Part model, mm, in its own coordinate system. A direction names the side the tool comes from. Round coordinates to 2 decimals unless told otherwise and drop trailing zeros. Loops run counter-clockwise (first coordinate to the right, second up) from the corner with the lowest first, then second, coordinate; pieces in that order, holes last.
from build123d import *

# Parameters (mm, degrees)
F0_W      = 50.8
F0_H      = 50.8
F1_DEPTH  = 50.8
F2_R      = 10.16
F3_DEPTH  = 2.54
F4_W      = 25.4
F4_H      = 14.759139
F5_DEPTH  = 2.54
F6_W      = 7.62
F6_H      = 2.876111
F7_DEPTH  = 5.08
F8_R      = 3.81
F9_DEPTH  = 5.08
F10_R     = 1.905
F11_DEPTH = 20.32
F12_R     = 1.778
F14_DEPTH = 53.34
F15_SIZE  = 1.27


with BuildPart() as f1:
    # F0 (on Front) → F1 (new body)
    with BuildSketch(Plane.XZ):
        with Locations((25.4, 25.4)):
            Rectangle(F0_W, F0_H)
    extrude(amount=F1_DEPTH)

    # F2 (on Right) → F3 (join)
    with BuildSketch(Plane.YZ):
        with Locations((-25.4, 35.56)):
            Circle(F2_R)
    extrude(amount=-F3_DEPTH)

    # F4 (on Right) → F5 (join)
    with BuildSketch(Plane.YZ):
        with Locations((-25.4, 10.40043)):
            Rectangle(F4_W, F4_H)
    extrude(amount=-F5_DEPTH)

    # F6 (on Right) → F7 (cut)
    with BuildSketch(Plane.YZ):
        with Locations((-19.05, 13.801944)):
            Rectangle(F6_W, F6_H)
        with Locations((-31.75, 13.801944)):
            Rectangle(F6_W, F6_H)
    extrude(amount=-F7_DEPTH, mode=Mode.SUBTRACT)

    # F8 (on Right) → F9 (join)
    with BuildSketch(Plane.YZ):
        with Locations((-25.4, 8.100861)):
            Circle(F8_R)
    extrude(amount=-F9_DEPTH)

    # F10 (on Right) → F11 (cut)
    with BuildSketch(Plane.YZ):
        with Locations((-31.771343, 38.1)):
            Circle(F10_R)
        with Locations((-19.028657, 38.1)):
            Circle(F10_R)
        with Locations((-19.028657, 33.02)):
            Circle(F10_R)
        with Locations((-31.771343, 33.02)):
            Circle(F10_R)
    extrude(amount=-F11_DEPTH, mode=Mode.SUBTRACT)

    # F12
    f12_edges = [f1.edges().sort_by_distance(p)[0] for p in [
        (0, -50.8, 25.4),
        (25.4, -50.8, 0),
        (50.8, -50.8, 25.4),
        (25.4, -50.8, 50.8),
        (50.8, -25.4, 50.8),
        (0, -25.4, 50.8),
        (25.4, 0, 50.8),
        (50.8, -25.4, 0),
        (50.8, 0, 25.4),
        (0, 0, 25.4),
        (25.4, 0, 0),
        (0, -25.4, 0),
    ]]
    fillet(f12_edges, radius=F12_R)

    # F13 (on Top) → F14 (join)
    with BuildSketch(Plane.XY):
        Polygon((18.288, -8.128), (8.128, -8.128), (8.128, -42.672), (42.672, -42.672), (42.672, -8.128), (32.512, -8.128), (32.512, -17.272), (18.288, -17.272), align=None)
    extrude(amount=F14_DEPTH)

    # F15
    f15_edges = [f1.edges().sort_by_distance(p)[0] for p in [
        (13.208, -8.128, 53.34),
        (8.128, -25.4, 53.34),
        (25.4, -42.672, 53.34),
        (42.672, -25.4, 53.34),
        (37.592, -8.128, 53.34),
        (32.512, -12.7, 53.34),
        (25.4, -17.272, 53.34),
        (18.288, -12.7, 53.34),
    ]]
    chamfer(f15_edges, length=F15_SIZE)


solid = f1.part
1) Tool access for faces 4 (the face through (-1, -38.1, 10)), 5 (the face through (25.73, -0.53, 0.51)), 6 (the face through (-1, -32, 15.24)): list every direction of +Z, -Z, +X, -X, +Y, -Y with a clear straight run to the whole face (end or side of a thin tool).
Values:
face 4: +Z, -Z, -X, -Y
face 5: -Z, +X, -X, +Y
face 6: -X
2) Slice it at D-D, the plane z = 47. Give the cut face in (x, y).
Values:
outline: (0, -49.02) arc R1.78 ccw to (1.78, -50.8) - (49.02, -50.8) arc R1.78 ccw to (50.8, -49.02) - (50.8, -1.78) arc R1.78 ccw to (49.02, 0) - (1.78, 0) arc R1.78 ccw to (0, -1.78) - close
3) Slice it at B-B, the plane y = -25.4. Give the cut face in (x, z).
Values:
outline: (-5.08, 4.29) - (-2.54, 4.29) - (-2.54, 3.02) - (0, 3.02) - (0, 1.78) arc R1.78 ccw to (1.78, 0) - (49.02, 0) arc R1.78 ccw to (50.8, 1.78) - (50.8, 49.02) arc R1.78 ccw to (49.02, 50.8) - (42.67, 50.8) - (42.67, 52.07) - (41.4, 53.34) - (9.4, 53.34) - (8.13, 52.07) - (8.13, 50.8) - (1.78, 50.8) arc R1.78 ccw to (0, 49.02) - (0, 45.72) - (-2.54, 45.72) - (-2.54, 25.4) - (0, 25.4) - (0, 17.78) - (-2.54, 17.78) - (-2.54, 11.91) - (-5.08, 11.91) - close
4) Wall check: line 1 along X through (y, z) = (-37, 36); line 2 along Y through (x, z) = (-1, 38). Give the ranges that are in metal, low to high.
Values:
line 1: x = 0 to 50.8
line 2: y = -35.26 to -33.67, -29.87 to -20.93, -17.13 to -15.54
5) Slice it at A-A, the plane z = 16.5. Give the cut face in (x, y), then the cut area to 3 significant figures.
Values:
outline: (-2.54, -38.1) - (0, -38.1) - (0, -49.02) arc R1.78 ccw to (1.78, -50.8) - (49.02, -50.8) arc R1.78 ccw to (50.8, -49.02) - (50.8, -1.78) arc R1.78 ccw to (49.02, 0) - (1.78, 0) arc R1.78 ccw to (0, -1.78) - (0, -12.7) - (-2.54, -12.7) - close
area: 2,640 mm2
6) Mould opens along Y. For faces 1 (the face through (-5.08, -25, 8)), 2 (the face through (25, -50.8, 26)), 3 (the face through (-1, -15.24, 14)) say: released by +Y, released by -Y, zero draft, split by the parting line, or undercut.
Values:
face 1: zero draft
face 2: released by -Y
face 3: undercut
7) Slice it at C-C, the plane x = 7. Give the cut face in (y, z).
Values:
outline: (-50.8, 1.78) arc R1.78 ccw to (-49.02, 0) - (-1.78, 0) arc R1.78 ccw to (0, 1.78) - (0, 49.02) arc R1.78 ccw to (-1.78, 50.8) - (-49.02, 50.8) arc R1.78 ccw to (-50.8, 49.02) - close
8) Drop flat-ended pins along their axis: pin 1 Ø5 at (y, z) = (-31.77, 38.1) entering from -X; pin 2 Ø1 at (x, z) = (24.5, 51.5) entering from +Y; pin 3 Ø0.9 at (y, z) = (-30, 14.5) entering from -X. Give the stop position or say it passes through.
Values:
pin 1: stops at x = -2.54
pin 2: stops at y = -17.27
pin 3: stops at x = 0
